```python
from build123d import *

# Parameters (mm, degrees)
IZIM1_R                     = 2.5
Y_KSEKLIK_EKSTR_ZYON1_DEPTH = 60
IZIM2_R                     = 2
Y_KSEKLIK_EKSTR_ZYON2_DEPTH = 2.5
KES_EKSTR_ZYON1_DEPTH       = 1
IZIM5_R                     = 1
KES_EKSTR_ZYON2_DEPTH       = 71


with BuildPart() as part:
    # Çizim1 → Yükseklik-Ekstrüzyon1 (new body)
    with BuildSketch(Plane.XY):
        Circle(IZIM1_R)
    extrude(amount=Y_KSEKLIK_EKSTR_ZYON1_DEPTH)

    # Çizim2 → Yükseklik-Ekstrüzyon2 (add)
    with BuildSketch(Plane.XY):
        Circle(IZIM2_R)
    extrude(amount=-Y_KSEKLIK_EKSTR_ZYON2_DEPTH)

    # Çizim4 → Kes-Ekstrüzyon1 (cut)
    with BuildSketch(Plane(origin=(0, 0, -2.5), x_dir=(-1, 0, 0), z_dir=(0, 0, -1))):
        with BuildLine():
            Line((-1.116104082, -1), (-1.732050808, -1))
            ThreePointArc((-1.732050808, -1), (-1.414213562, -1.414213562), (-1, -1.732050808))
            Line((-1, -1.732050808), (-1, -1.116104082))
            ThreePointArc((-1, -1.116104082), (-1.059643412, -1.059643412), (-1.116104082, -1))
        make_face()
        with BuildLine():
            Line((-0.466574488, -1.424077445), (-1, -1.732050808))
            ThreePointArc((-1, -1.732050808), (-0.51763809, -1.931851653), (0, -2))
            Line((0, -2), (-0.307973363, -1.466574488))
            ThreePointArc((-0.307973363, -1.466574488), (-0.387856408, -1.44749982), (-0.466574488, -1.424077445))
        make_face()
        with BuildLine():
            Line((0.307973363, -1.466574488), (0, -2))
            ThreePointArc((0, -2), (0.51763809, -1.931851653), (1, -1.732050808))
            Line((1, -1.732050808), (0.466574488, -1.424077445))
            ThreePointArc((0.466574488, -1.424077445), (0.387856408, -1.44749982), (0.307973363, -1.466574488))
        make_face()
        with BuildLine():
            Line((1, -1.116104082), (1, -1.732050808))
            ThreePointArc((1, -1.732050808), (1.414213562, -1.414213562), (1.732050808, -1))
            Line((1.732050808, -1), (1.116104082, -1))
            ThreePointArc((1.116104082, -1), (1.059643412, -1.059643412), (1, -1.116104082))
        make_face()
        with BuildLine():
            ThreePointArc((1.732050808, -1), (1.931851653, -0.51763809), (2, 0))
            Line((2, 0), (1.466574488, -0.307973363))
            ThreePointArc((1.466574488, -0.307973363), (1.44749982, -0.387856408), (1.424077445, -0.466574488))
            Line((1.424077445, -0.466574488), (1.732050808, -1))
        make_face()
        with BuildLine():
            ThreePointArc((2, 0), (1.931851653, 0.51763809), (1.732050808, 1))
            Line((1.732050808, 1), (1.424077445, 0.466574488))
            ThreePointArc((1.424077445, 0.466574488), (1.44749982, 0.387856408), (1.466574488, 0.307973363))
            Line((1.466574488, 0.307973363), (2, 0))
        make_face()
        with BuildLine():
            ThreePointArc((1.732050808, 1), (1.414213562, 1.414213562), (1, 1.732050808))
            Line((1, 1.732050808), (1, 1.116104082))
            ThreePointArc((1, 1.116104082), (1.059643412, 1.059643412), (1.116104082, 1))
            Line((1.116104082, 1), (1.732050808, 1))
        make_face()
        with BuildLine():
            ThreePointArc((1, 1.732050808), (0.51763809, 1.931851653), (0, 2))
            Line((0, 2), (0.307973363, 1.466574488))
            ThreePointArc((0.307973363, 1.466574488), (0.387856408, 1.44749982), (0.466574488, 1.424077445))
            Line((0.466574488, 1.424077445), (1, 1.732050808))
        make_face()
        with BuildLine():
            ThreePointArc((0, 2), (-0.51763809, 1.931851653), (-1, 1.732050808))
            Line((-1, 1.732050808), (-0.466574488, 1.424077445))
            ThreePointArc((-0.466574488, 1.424077445), (-0.387856408, 1.44749982), (-0.307973363, 1.466574488))
            Line((-0.307973363, 1.466574488), (0, 2))
        make_face()
        with BuildLine():
            ThreePointArc((-1, 1.732050808), (-1.414213562, 1.414213562), (-1.732050808, 1))
            Line((-1.732050808, 1), (-1.116104082, 1))
            ThreePointArc((-1.116104082, 1), (-1.059643412, 1.059643412), (-1, 1.116104082))
            Line((-1, 1.116104082), (-1, 1.732050808))
        make_face()
        with BuildLine():
            Line((-1.424077445, 0.466574488), (-1.732050808, 1))
            ThreePointArc((-1.732050808, 1), (-1.931851653, 0.51763809), (-2, 0))
            Line((-2, 0), (-1.466574488, 0.307973363))
            ThreePointArc((-1.466574488, 0.307973363), (-1.44749982, 0.387856408), (-1.424077445, 0.466574488))
        make_face()
        with BuildLine():
            Line((-1.466574488, -0.307973363), (-2, 0))
            ThreePointArc((-2, 0), (-1.931851653, -0.51763809), (-1.732050808, -1))
            Line((-1.732050808, -1), (-1.424077445, -0.466574488))
            ThreePointArc((-1.424077445, -0.466574488), (-1.44749982, -0.387856408), (-1.466574488, -0.307973363))
        make_face()
    extrude(amount=-KES_EKSTR_ZYON1_DEPTH, mode=Mode.SUBTRACT)

    # Çizim5 → Kes-Ekstrüzyon2 (cut)
    with BuildSketch(Plane(origin=(0, 0, -2.5), x_dir=(-1, 0, 0), z_dir=(0, 0, -1))):
        Circle(IZIM5_R)
    extrude(amount=-KES_EKSTR_ZYON2_DEPTH, mode=Mode.SUBTRACT)


solid = part.part
```
Here's how the part is built. I have some questions about the finished solid (model axes, mm). A direction names the side the tool comes from. Give positions to 0.01 mm unless a question says otherwise; leave off trailing zeros. Loops run counter-clockwise (first coordinate to the right, second up) from the corner with the lowest first, then second, coordinate; pieces in that order, holes last. Notation, with made-up numbers: (-39, 26.5) -> (2, 26.5) arc R32 cw to (2, 55.5) -> close; hole circle Ø2 at (46, 36.5). An arc over 180 degrees is marked (long way). Use one line per item in the form item = value. Start each with the question number.
1) Please list where these lines run through material, in increasing order: line 1 along Y through (x, z) = (0, 19); line 2 along Z through (x, y) = (-0.35, 1.8); line 3 along Z through (x, y) = (0.35, -2.25).
2) For P1, Ø0.5, axis at y = -1.5, z = -2, coming from the -X side; P2, Ø0.7, axis at x = -1.5, z = -2, coming from the +Y side; P3, Ø0.8, axis at x = 1.5, y = 1.5, coming from the -Z side, each with a flat end and sliding along its axis, tell me the tip position at first contact or that it passes through.
3) Thinking about a two-plate mould opening in Y: for faces 3 (the face through (0, -1, 28)), 4 (the face through (-0.54, -2.44, 29.58)), 5 (the face through (-1, 2, 0)), which applies, +Y half, -Y half, draft (parallel to the pull), parting line (faces both ways), or undercut?
4) Which directions (+Z, -Z, +X, -X, +Y, -Y) give clear straight access to the entire face, cutting with the end or side of a thin tool? Please do faces 1 (the face through (1.847, -0.766, -0.74)), 2 (the face through (-0.9, 0.9, -2.5)).
5) Imagine slicing it at A-A (z = 14). Please give me the cut outline in (x, y), then the cut area to 3 significant figures.
Check values:
q1.line_1 = -2.5 to -1, 1 to 2.5
q1.line_2 = -1.5 to 60
q1.line_3 = 0 to 60
q2.P1 = -1
q2.P2 = 1
q2.P3 = -1.5
q3.face_3 = undercut
q3.face_4 = parting line
q3.face_5 = draft
q4.face_1 = -Z
q4.face_2 = -Z, +X, -X, +Y, -Y
q5.outline = circle Ø5 at (0, 0); hole circle Ø2 at (0, 0)
q5.area = 16.5 mm^2
